Design review of the part built by this model. Coordinates are the model's own, in mm. Face numbers are marked on the shaded views. A direction names the side the tool comes from. Round coordinates to 2 decimals unless told otherwise and drop trailing zeros. Loops run counter-clockwise (first coordinate to the right, second up) from the corner with the lowest first, then second, coordinate; pieces in that order, holes last. Notation, with made-up numbers: M 40.25,-18.5 L 67.25,-18.5 A20 ccw 67.25,8.5 Z; hole C 8,10.25 d3. An arc over 180 degrees is marked long. Use a Markdown table: item, result.
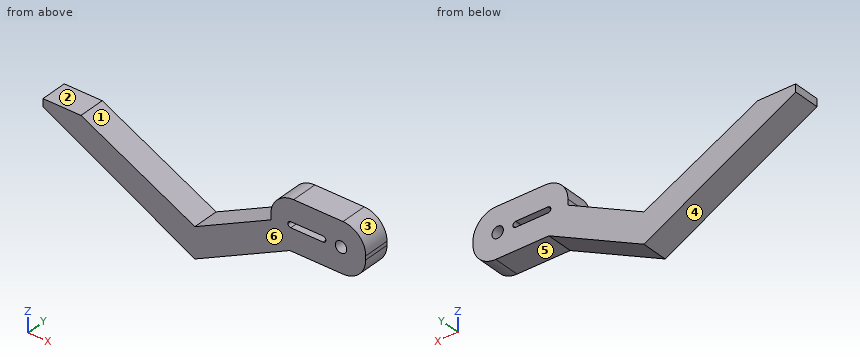
from build123d import *

# Parameters (mm, degrees)
SKETCH1_W                = 25
SKETCH1_H                = 13
BOSS_EXTRUDE1_DEPTH      = 7
F_3_0_3_DIAMETER_HOLE3_D = 3
FILLET7_R                = 6
CUT_EXTRUDE1_DEPTH       = 52.019604075
FILLET8_R                = 0.75


with BuildPart() as part:
    # Sketch1 → Boss-Extrude1 (new body)
    with BuildSketch(Plane(origin=(0, 0, 0), x_dir=(1, 0, 0), z_dir=(0, 1, 0))):
        Polygon((-40, 0), (-30, 0), (0, 15), (20, 5), (20, 10.5), (25, 10.5), (0, 23), (-40, 2), align=None)
        with Locations((32.5, 4)):
            Rectangle(SKETCH1_W, SKETCH1_H)
    extrude(amount=BOSS_EXTRUDE1_DEPTH)

    # Ø3.0 (3) Diameter Hole3 (through all)
    with Locations(Plane(origin=(0, 7, 0), x_dir=(1, 0, 0), z_dir=(0, 1, 0))):
        with Locations((38.5, 4)):
            Hole(F_3_0_3_DIAMETER_HOLE3_D / 2)

    # Fillet7
    fillet7_edges = [part.edges().sort_by_distance(p)[0] for p in [
        (20, 3.5, 2.5),
        (45, 3.5, 2.5),
        (45, 3.5, -10.5),
    ]]
    fillet(fillet7_edges, radius=FILLET7_R)

    # Sketch11 → Cut-Extrude1 (cut, through all)
    with BuildSketch(Plane(origin=(0, 7, 0), x_dir=(1, 0, 0), z_dir=(0, 1, 0))):
        Polygon((24.5, 4), (24.5, 3.25), (34.5, 3.25), (34.5, 4.75), (24.5, 4.75), align=None)
    extrude(amount=-CUT_EXTRUDE1_DEPTH, mode=Mode.SUBTRACT)

    # Fillet8
    fillet8_edges = [part.edges().sort_by_distance(p)[0] for p in [
        (34.5, 3.5, -3.25),
        (34.5, 3.5, -4.75),
        (24.5, 3.5, -4.75),
        (24.5, 3.5, -3.25),
    ]]
    fillet(fillet8_edges, radius=FILLET8_R - 0.0001)  # a hair under: the kernel refuses the full size


solid = part.part
1. The part is to be moulded in two halves that separate along X. For the marked faces 1, 2, 3 and 4, say which applies: pulls with the +X half, pulls with the -X half, needs draft (parallel to the pull), parting line crosses it, or undercut.
Check values:
| item | result |
|---|---|
| face 1 | undercut |
| face 2 | needs draft |
| face 3 | pulls with the +X half |
| face 4 | pulls with the -X half |
2. Take a section at D-D on z = -7.75. Give the boundary of the cut face in (x, y), and give its area (3 significant figures).
Check values:
| item | result |
|---|---|
| outline | M -29.05,0 L -14.5,0 L -14.5,7 L -29.05,7 Z; M 14.5,0 L 44.04,0 L 44.04,7 L 14.5,7 Z |
| area | 309 mm² |
3. Take a section at A-A on z = -12.5. Give the boundary of the cut face in (x, y), and give its area (3 significant figures).
Check values:
| item | result |
|---|---|
| outline | M -20,0 L -5,0 L -5,7 L -20,7 Z; M 5,0 L 21,0 L 21,7 L 5,7 Z |
| area | 217 mm² |
4. Machinability: for the marked faces 5 and 6, which of the approach directions +Z, -Z, +X, -X, +Y, -Y give a long, thin tool a straight path to every point of the face, cutting with its end or side? Answer none if there is none.
Check values:
| item | result |
|---|---|
| face 5 | -Z, +X, +Y, -Y |
| face 6 | +Z, -Z, +X, -X, -Y |
5. Insertion check: pin 1 (4 mm diameter, centred on y = 3, z = -17.5, fed in from +X); pin 2 (0.8 mm diameter, centred on y = 2, z = -4.5, fed in from -X); pin 3 (3.5 mm diameter, centred on x = -37, y = 4, fed in from +Z). Each pin has a flat end and moves straight along its axis. Give the tip position at first contact, or say it passes through.
Check values:
| item | result |
|---|---|
| pin 1 | stops at x = 15 |
| pin 2 | stops at x = -36 |
| pin 3 | stops at z = 0 |
6. Wall thickness on line 1 along Z through (x, y) = (38.5, 4.5); line 2 along Z through (x, y) = (29.5, 5.25); line 3 along X through (y, z) = (5.5, -1.75): over which ranges is each line inside the solid? List them lowest first. Write a range as from..to.
Check values:
| item | result |
|---|---|
| line 1 | z = -10.5..-5.5, -2.5..2.5 |
| line 2 | z = -10.5..-4.75, -3.25..2.5 |
| line 3 | x = -40..-26.5, 20.26..44.74 |
7. Take a section at B-B on y = 1. Count the separate pieces of the cut face and the enclosed holes in it, and give its area (3 significant figures).
Check values:
| item | result |
|---|---|
| separate pieces | 1 |
| enclosed holes | 2 |
| area | 721 mm² |
8. Take a section at C-C on x = -2. Give the boundary of the cut face in (y, z), and give its area (4 significant figures).
Check values:
| item | result |
|---|---|
| outline | M 0,-21.95 L 7,-21.95 L 7,-14 L 0,-14 Z |
| area | 55.65 mm² |
